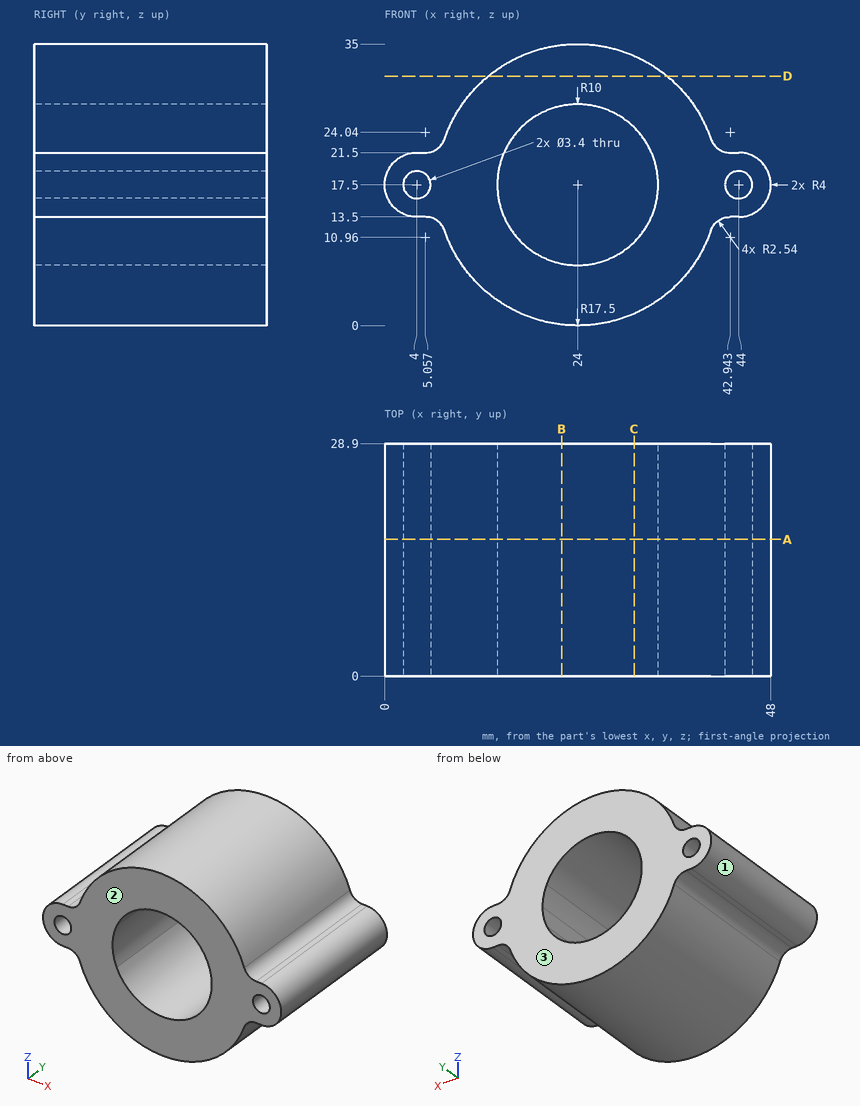
Study the drawing (mm; zero at the part's minimum x, y, z) and answer. Coordinates: 2 decimals unless noted, no trailing zeros. Write each loop counter-clockwise with the first axis right and the second up, starting at its lowest first coordinate (ties: lowest second). Pieces come first, ordered by that corner, then holes. Notation, with made-up numbers: (16, -32.5) -> (45, -32.5) arc R14 ccw to (45, -11.5) -> close; hole circle Ø2 at (8, 3.25). An arc over 180 degrees is marked (long way). Write item = value, one per line.
(1) Straight lines are drawn through the part: L1, parallel to X at y = 9.25, z = 17.5; L2, parallel to Z at x = 44, y = 23; L3, parallel to X at y = 2.75, z = 24.5. For each, find the intervals that lie inside material, in ascending order. Write a range as from..to.
From the geometry:
L1 = 0..2.3, 5.7..14, 34..42.3, 45.7..48
L2 = 13.5..15.8, 19.2..21.5
L3 = 7.96..16.86, 31.14..40.04
(2) For a pull along Y with two mould halves and no side action, classify the marked faces 1, 2 and 3 as +Y half, -Y half, draft (parallel to the pull), parting line (faces both ways), or undercut.
From the geometry:
face_1 = draft
face_2 = -Y half
face_3 = +Y half
(3) Section A-A on y = 17 is taken. Write down the section's boundary in (x, z) (1 decimal).
From the geometry:
outline = (4, 13.5) -> (5.1, 13.5) arc R2.5 cw to (7.5, 11.8) arc R17.5 ccw to (40.5, 11.8) arc R2.5 cw to (42.9, 13.5) -> (44, 13.5) arc R4 ccw to (44, 21.5) -> (42.9, 21.5) arc R2.5 cw to (40.5, 23.2) arc R17.5 ccw to (7.5, 23.2) arc R2.5 cw to (5.1, 21.5) -> (4, 21.5) arc R4 ccw to start; hole circle Ø3.4 at (4, 17.5); hole circle Ø20 at (24, 17.5); hole circle Ø3.4 at (44, 17.5)
(4) Section C-C on x = 31 is taken. Write down the section's boundary in (y, z).
From the geometry:
outline = (0, 1.46) -> (28.9, 1.46) -> (28.9, 10.36) -> (0, 10.36) -> close; (0, 24.64) -> (28.9, 24.64) -> (28.9, 33.54) -> (0, 33.54) -> close
(5) Given pin 1 Ø1.2 at (x, y) = (43.5, 13) entering from +Z; pin 2 Ø1 at (y, z) = (9.5, 9) entering from +X; pin 3 Ø6 at (x, z) = (41.5, 31.5) entering from +Y (1 decimal); pin 4 Ø0.8 at (x, y) = (4.5, 9.5) entering from -Z, each flat-ended and moving along its own axis, determine where each tip first touches the part or whether it passes through.
From the geometry:
pin_1 = 21.5
pin_2 = 39.56
pin_3 = through
pin_4 = 13.5
(6) Section B-B on x = 22 is taken. Write down the section's boundary in (y, z) (1 decimal).
From the geometry:
outline = (0, 0.1) -> (28.9, 0.1) -> (28.9, 7.7) -> (0, 7.7) -> close; (0, 27.3) -> (28.9, 27.3) -> (28.9, 34.9) -> (0, 34.9) -> close
(7) Section D-D on z = 31 is taken. Write down the section's boundary in (x, y), plus the area to 3 significant figures.
From the geometry:
outline = (12.86, 0) -> (35.14, 0) -> (35.14, 28.9) -> (12.86, 28.9) -> close
area = 644 mm2
